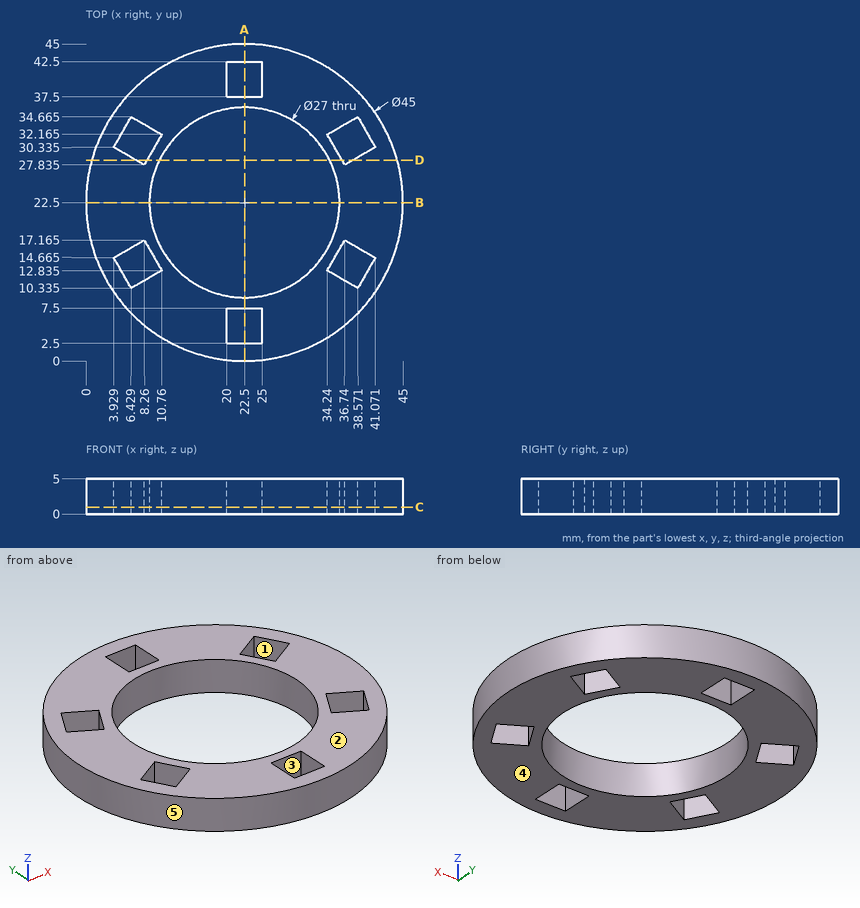
Design review of the part shown in the three views and the two pictorial views. Dimensions are in mm from the part's minimum x, y and z. A direction names the side the tool comes from. Give positions to 0.01 mm unless a question says otherwise; leave off trailing zeros. Loops run counter-clockwise (first coordinate to the right, second up) from the corner with the lowest first, then second, coordinate; pieces in that order, holes last. Notation, with made-up numbers: (-39.5, -25.75) -> (-28.5, -25.75) arc R12 ccw to (-28.5, -6.75) -> close; hole circle Ø6 at (42.25, 30.25). An arc over 180 degrees is marked (long way). One line per question, with ' | ' between items.
1) We need section A-A (x = 22.5). Write out the cut boundary in (y, z).
Resolved:
outline: (0, 0) -> (2.5, 0) -> (2.5, 5) -> (0, 5) -> close; (7.5, 0) -> (9, 0) -> (9, 5) -> (7.5, 5) -> close; (36, 0) -> (37.5, 0) -> (37.5, 5) -> (36, 5) -> close; (42.5, 0) -> (45, 0) -> (45, 5) -> (42.5, 5) -> close
2) The part is to be moulded in two halves that separate along X. For the marked faces 3, 4 and 5, say which applies: +X half, -X half, draft (parallel to the pull), parting line (faces both ways), or undercut.
Resolved:
face 3: undercut | face 4: draft | face 5: parting line
3) For the marked faces 1 and 2, list the 3-axis set-ups (+Z, -Z, +X, -X, +Y, -Y) from which the entire face can be reached by the end or side of a thin tool; tool diameter is ignored.
Resolved:
face 1: +Z, -Z | face 2: +Z, +X, -X, +Y, -Y
4) We need section B-B (y = 22.5). Write out the cut boundary in (x, z).
Resolved:
outline: (0, 0) -> (9, 0) -> (9, 5) -> (0, 5) -> close; (36, 0) -> (45, 0) -> (45, 5) -> (36, 5) -> close
5) To check wall thickness, follow probe 1 along Y at (x, z) = (22.5, 2.2); probe 2 along X at (y, z) = (4.5, 1.25); probe 3 along Y at (x, z) = (7.5, 1.8) (1 decimal). State the ranges of each line that lie inside material, in increasing order.
Resolved:
probe 1: y = 0 to 2.5, 7.5 to 9, 36 to 37.5, 42.5 to 45 | probe 2: x = 9 to 20, 25 to 36 | probe 3: y = 5.7 to 11, 16.7 to 28.3, 34 to 39.3
6) Insertion check: pin 1 Ø2.5 at (y, z) = (4, 1.5) entering from +X (1 decimal); pin 2 Ø3 at (x, z) = (12.5, 4.5) entering from +Y; pin 3 Ø1.5 at (x, z) = (23.5, 3.5) entering from -Y; pin 4 Ø16 at (x, y) = (22.5, 22.5) entering from -Z. Each pin has a flat end and moves straight along its axis. Give the tip position at first contact, or say it passes through.
Resolved:
pin 1: stops at x = 36.9 | pin 2: stops at y = 43.33 | pin 3: stops at y = 0 | pin 4: passes through
7) We need section C-C (z = 1). Write out the cut boundary in (x, y) (1 decimal).
Resolved:
outline: circle Ø45 at (22.5, 22.5); hole (3.9, 14.7) -> (6.4, 10.3) -> (10.8, 12.8) -> (8.3, 17.2) -> close; hole (3.9, 30.3) -> (8.3, 27.8) -> (10.8, 32.2) -> (6.4, 34.7) -> close; hole circle Ø27 at (22.5, 22.5); hole (20, 2.5) -> (25, 2.5) -> (25, 7.5) -> (20, 7.5) -> close; hole (20, 37.5) -> (25, 37.5) -> (25, 42.5) -> (20, 42.5) -> close; hole (34.2, 12.8) -> (38.6, 10.3) -> (41.1, 14.7) -> (36.7, 17.2) -> close; hole (34.2, 32.2) -> (36.7, 27.8) -> (41.1, 30.3) -> (38.6, 34.7) -> close
8) We need section D-D (y = 28.5). Write out the cut boundary in (x, z) (1 decimal).
Resolved:
outline: (0.8, 0) -> (7.1, 0) -> (7.1, 5) -> (0.8, 5) -> close; (8.6, 0) -> (10.4, 0) -> (10.4, 5) -> (8.6, 5) -> close; (34.6, 0) -> (36.4, 0) -> (36.4, 5) -> (34.6, 5) -> close; (37.9, 0) -> (44.2, 0) -> (44.2, 5) -> (37.9, 5) -> close
